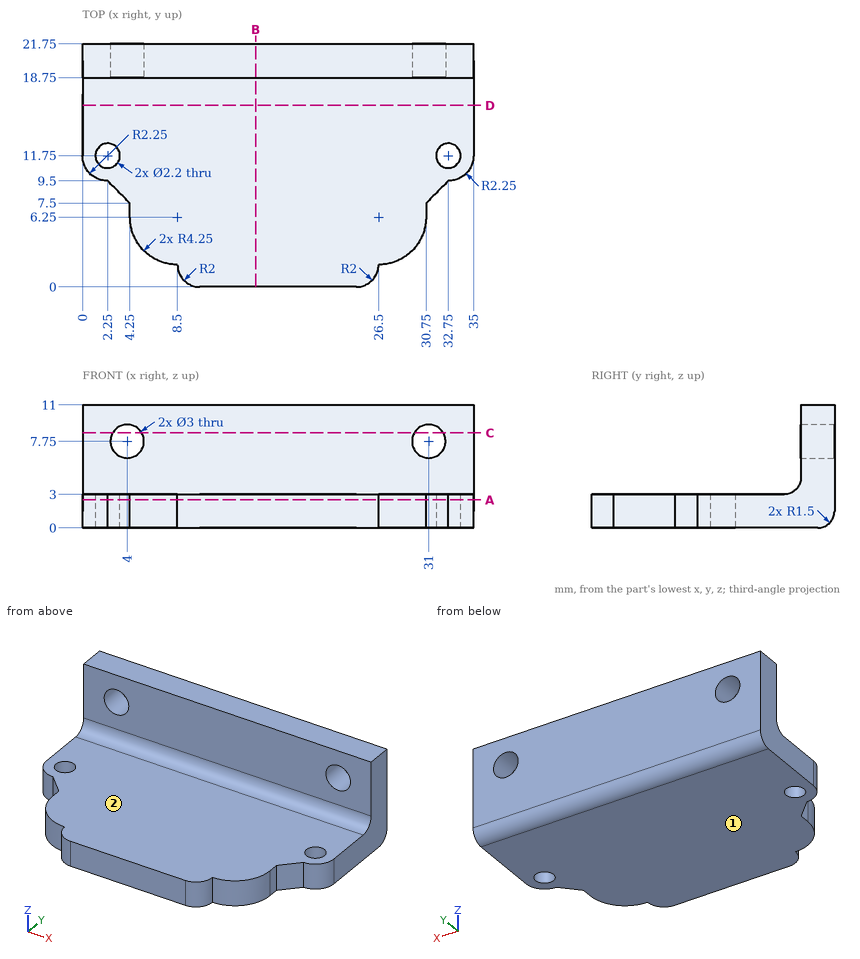
Here's the drawing with two shaded views (mm, measured from the low corner). I have some questions. A direction names the side the tool comes from. Give positions to 0.01 mm unless a question says otherwise; leave off trailing zeros. Order: outer loops, then holes, each group sorted by start corner. A loop starts at its lowest first (then second) coordinate and runs counter-clockwise, first axis right, second up. Notation, with made-up numbers: (34.25, 48) - (53.25, 48) arc R19 cw to (53.25, 80) - close; hole circle Ø10 at (-25, 61.25). An arc over 180 degrees is marked (long way). Use a Markdown table: item, result. Add a question column.
Q1. If we section it at C-C on z = 8.5: Write out the boundary of the cut face in (x, y), plus the area to 3 significant figures.
Q2. If we section it at A-A on z = 2.5: Count the separate pieces of the cut face and the enclosed holes in it, plus the area to 3 significant figures.
Q3. On a 3-axis mill with a long thin cutter (end or side, diameter ignored), from which of +Z, -Z, +X, -X, +Y, -Y can I reach the whole of each face in a straight line? I mean the marked faces 1 and 2. Say none if no direction works.
Q4. If we section it at B-B on x = 15.5: Write out the boundary of the cut face in (y, z).
Q5. If we section it at D-D on y = 16.25: Write out the boundary of the cut face in (x, z).
Q6. I'm going to push flat-ended pins straight in: pin 1 (4 mm diameter, centred on x = 31, z = 7.75, fed in from +Y); pin 2 (3 mm diameter, centred on x = 11, z = 6.5, fed in from -Y); pin 3 (2.5 mm diameter, centred on x = 32.75, y = 11.75, fed in from +Z); pin 4 (0.6 mm diameter, centred on y = 6.5, z = 1, fed in from +X). Where does each tip first touch, or does it pass through?
Q7. Please list where these lines run through material, in increasing order: line 1 along X through (y, z) = (19.95, 7.75); line 2 along Y through (x, z) = (32.75, 2.35); line 3 along Y through (x, z) = (32.5, 9.5).
Answers follow:
| question | item | result |
|---|---|---|
| 1 | outline | (0, 18.75) - (2.7, 18.75) - (2.7, 21.75) - (0, 21.75) - close; (5.3, 18.75) - (29.7, 18.75) - (29.7, 21.75) - (5.3, 21.75) - close; (32.3, 18.75) - (35, 18.75) - (35, 21.75) - (32.3, 21.75) - close |
| 1 | area | 89.4 mm^2 |
| 2 | separate pieces | 1 |
| 2 | enclosed holes | 2 |
| 2 | area | 648 mm^2 |
| 3 | face 1 | -Z, +X, -X, +Y, -Y |
| 3 | face 2 | +Z, +X, -X, -Y |
| 4 | outline | (0, 0) - (20.25, 0) arc R1.5 ccw to (21.75, 1.5) - (21.75, 11) - (18.75, 11) - (18.75, 4.5) arc R1.5 cw to (17.25, 3) - (0, 3) - close |
| 5 | outline | (0, 0) - (35, 0) - (35, 3) - (0, 3) - close |
| 6 | pin 1 | stops at y = 21.75 |
| 6 | pin 2 | stops at y = 18.75 |
| 6 | pin 3 | stops at z = 3 |
| 6 | pin 4 | stops at x = 30.75 |
| 7 | line 1 | x = 0 to 2.5, 5.5 to 29.5, 32.5 to 35 |
| 7 | line 2 | y = 9.5 to 10.65, 12.85 to 21.75 |
| 7 | line 3 | y = 18.75 to 21.75 |
